Here's how the part is built. I have some questions about the finished solid (model axes, mm). A direction names the side the tool comes from. Round coordinates to 2 decimals unless told otherwise and drop trailing zeros. Loops run counter-clockwise (first coordinate to the right, second up) from the corner with the lowest first, then second, coordinate; pieces in that order, holes last. Notation, with made-up numbers: (15, -27.75) - (62, -27.75) arc R28 ccw to (62, 10.25) - close; hole circle Ø6 at (48, -22). An arc over 180 degrees is marked (long way). Answer as a JSON object with one key per item and string values. Group by question number.
1) If I drill on line 1 along X through (y, z) = (0, -2.25); line 2 along Y through (x, z) = (8.75, -0.9); line 3 along Y through (x, z) = (7.25, -0.5), over which ranges is the centre line in solid material (lowest first)? Write a range as [from, to].
2) Which directions (+Z, -Z, +X, -X, +Y, -Y) give clear straight access to the entire face, cutting with the end or side of a thin tool? Please do faces 4 (the face through (0, 9, -2)), 5 (the face through (0, -9, -2)), 6 (the face through (-7.5, 0, -4.1)), 7 (the face through (-11, 3, -3)), 8 (the face through (11, -3, -3)).
3) I want a section at A-A, the plane z = -2.5. Please give me the cut outline in (x, y), then the cut area to 3 significant figures.
4) I want a section at D-D, the plane y = -12.25. Please give me the cut outline in (x, z).
5) Will these pins go through, and if not, where does the flat tip stop? P1, Ø9, axis at x = 5, y = 9.5, coming from the -Z side; P2, Ø3, axis at x = -7.95, y = -7.95, coming from the -Z side; P3, Ø2, axis at x = 6, z = -1.5, coming from the +Y side.
6) I want a section at B-B, the plane z = -4. Please give me the cut outline in (x, y), then the cut area to 3 significant figures.
7) If we mould it in two halves opening along Y, with no side actions, what happens to faces 1 (the face through (-7.378, -6.846, -0.986)), 2 (the face through (-7, 3, 0)), 3 (the face through (-10, -3, -3))? For each: pulls with the +Y half, pulls with the -Y half, needs draft (parallel to the pull), parting line crosses it, or undercut.
8) I want a section at C-C, the plane x = 0. Please give me the cut outline in (y, z).
from build123d import *

# Parameters (mm, degrees)
F0_R     = 5
F2_DEPTH = 3.2
F0_R_2   = 1.25
F3_DEPTH = 2
F4_DEPTH = 5
F5_SIZE  = 2
F6_ANGLE = 180


with BuildPart() as f2:
    # F0 (on Top) → F2 (new body)
    with BuildSketch(Plane.XY):
        with BuildLine():
            ThreePointArc((7.5, 0), (7.341797347, 1.5323223277), (6.8738635424, 3))
            ThreePointArc((6.8738635424, 3), (0, 7.5), (-6.8738635424, 3))
            ThreePointArc((-6.8738635424, 3), (-7.5, 0), (-6.8738635424, -3))
            ThreePointArc((-6.8738635424, -3), (0, -7.5), (6.8738635424, -3))
            ThreePointArc((6.8738635424, -3), (7.341797347, -1.5323223277), (7.5, 0))
        make_face()
        Circle(F0_R, mode=Mode.SUBTRACT)
    extrude(amount=F2_DEPTH)

    # F0 (on Top) → F3 (join)
    with BuildSketch(Plane.XY):
        with BuildLine():
            Line((6.8738635424, 3), (14.1862609591, 3))
            ThreePointArc((14.1862609591, 3), (0, 14.5), (-14.1862609591, 3))
            Line((-14.1862609591, 3), (-6.8738635424, 3))
            ThreePointArc((-6.8738635424, 3), (0, 7.5), (6.8738635424, 3))
        make_face()
        with Locations((-7.9549512883, 7.9549512883)):
            Circle(F0_R_2, mode=Mode.SUBTRACT)
        with Locations((7.9549512883, 7.9549512883)):
            Circle(F0_R_2, mode=Mode.SUBTRACT)
        with BuildLine():
            ThreePointArc((-14.1862609591, -3), (0, -14.5), (14.1862609591, -3))
            Line((14.1862609591, -3), (6.8738635424, -3))
            ThreePointArc((6.8738635424, -3), (0, -7.5), (-6.8738635424, -3))
            Line((-6.8738635424, -3), (-14.1862609591, -3))
        make_face()
        with Locations((-7.9549512883, -7.9549512883)):
            Circle(F0_R_2, mode=Mode.SUBTRACT)
        with Locations((7.9549512883, -7.9549512883)):
            Circle(F0_R_2, mode=Mode.SUBTRACT)
    extrude(amount=F3_DEPTH)

    # F0 (on Top) → F4 (join)
    with BuildSketch(Plane.XY):
        with BuildLine():
            Line((-6.8738635424, 3), (-14.1862609591, 3))
            ThreePointArc((-14.1862609591, 3), (-14.5, 0), (-14.1862609591, -3))
            Line((-14.1862609591, -3), (-6.8738635424, -3))
            ThreePointArc((-6.8738635424, -3), (-7.5, 0), (-6.8738635424, 3))
        make_face()
        with BuildLine():
            ThreePointArc((14.1862609591, -3), (14.4213519461, -1.508180376), (14.5, 0))
            ThreePointArc((14.5, 0), (14.4213519461, 1.508180376), (14.1862609591, 3))
            Line((14.1862609591, 3), (6.8738635424, 3))
            ThreePointArc((6.8738635424, 3), (7.341797347, 1.5323223277), (7.5, 0))
            ThreePointArc((7.5, 0), (7.341797347, -1.5323223277), (6.8738635424, -3))
            Line((6.8738635424, -3), (14.1862609591, -3))
        make_face()
    extrude(amount=F4_DEPTH)

    # F5
    f5_edges = [f2.edges().sort_by_distance(p)[0] for p in [
        (-5, 0, 0),
    ]]
    chamfer(f5_edges, length=F5_SIZE)


with BuildPart() as f2_1:
    # F6: moved
    add(f2.part.rotate(Axis((20.4745046794, 0, 0), (1, 0, 0)), F6_ANGLE))


solid = f2_1.part
Outcome:
{
 "1": {"line 1": "[-14.5, -5], [5, 14.5]", "line 2": "[-11.56, -8.92], [-6.99, 6.99], [8.92, 11.56]", "line 3": "[-12.56, -8.99], [-6.92, 6.92], [8.99, 12.56]"},
 "2": {"face 4": "-Z, +Y", "face 5": "-Z, -Y", "face 6": "-Z", "face 7": "-Z, -X, +Y", "face 8": "-Z, +X, -Y"},
 "3": {"outline": "(-14.19, -3) - (-6.87, -3) arc R7.5 ccw to (6.87, -3) - (14.19, -3) arc R14.5 ccw to (14.19, 3) - (6.87, 3) arc R7.5 ccw to (-6.87, 3) - (-14.19, 3) arc R14.5 ccw to start; hole circle Ø10 at (0, 0)", "area": "183 mm^2"},
 "4": {"outline": "(-7.76, -2) - (7.76, -2) - (7.76, 0) - (-7.76, 0) - close"},
 "5": {"P1": "z = -3.2", "P2": "z = -2", "P3": "y = 13.61"},
 "6": {"outline": "(-14.19, -3) - (-6.87, -3) arc R7.5 cw to (-6.87, 3) - (-14.19, 3) arc R14.5 ccw to start; (6.87, -3) - (14.19, -3) arc R14.5 ccw to (14.19, 3) - (6.87, 3) arc R7.5 cw to start", "area": "85.2 mm^2"},
 "7": {"face 1": "undercut", "face 2": "needs draft", "face 3": "pulls with the -Y half"},
 "8": {"outline": "(-14.5, -2) - (-7.5, -2) - (-7.5, -3.2) - (-5, -3.2) - (-5, -2) - (-7, 0) - (-14.5, 0) - close; (5, -3.2) - (7.5, -3.2) - (7.5, -2) - (14.5, -2) - (14.5, 0) - (7, 0) - (5, -2) - close"}
}
